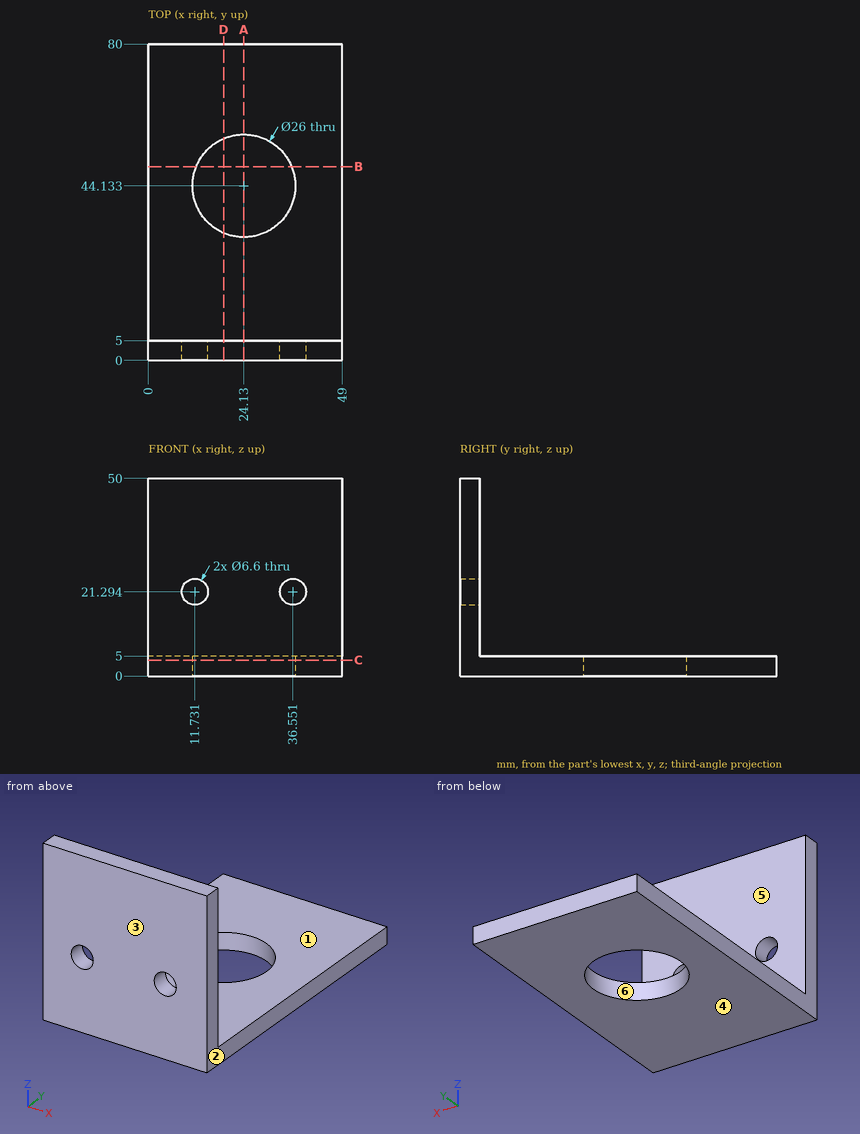
Part print with two shaded views. Sizes in mm from the minimum x, y, z corner. A direction names the side the tool comes from. Round coordinates to 2 decimals unless told otherwise and drop trailing zeros. Order: outer loops, then holes, each group sorted by start corner. A loop starts at its lowest first (then second) coordinate and runs counter-clockwise, first axis right, second up.
(1) Band-saw the part on D-D (x = 19). List the corners of the cut face in (y, z).
(2) Band-saw the part on B-B (y = 49). List the corners of the cut face in (x, z) (1 decimal).
(3) 3-axis set-ups, long thin cutter, end or side, ignore diameter. For the marked faces 1 and 2: which of +Z, -Z, +X, -X, +Y, -Y reach the whole face in a straight line?
(4) Pull direction Y, two halves, no side cores. Call the marked faces 3, 4, 5 and 6: released by +Y, released by -Y, zero draft, split by the parting line, or undercut.
(5) Pin check, flat tips, straight feed: pin 1 (14.5 mm diameter, centred on x = 17.5, y = 31, fed in from +Z); pin 2 (7.5 mm diameter, centred on x = 11.73, z = 21.29, fed in from +Y). Stop position of each tip, or through.
(6) Band-saw the part on C-C (z = 4). List the corners of the cut face in (x, y), then the cut area to 3 significant figures.
(7) Drill centre lines: line 1 (Y direction, x = 24, z = 3); line 2 (Z direction, x = 26, y = 14). Where is each one in solid material? Low to high.
(8) Band-saw the part on A-A (x = 24.13). List the corners of the cut face in (y, z), then the cut area to 3 significant figures.
Verdict:
1. outline: (0, 0) - (32.19, 0) - (32.19, 5) - (5, 5) - (5, 50) - (0, 50) - close; (56.08, 0) - (80, 0) - (80, 5) - (56.08, 5) - close
2. outline: (0, 0) - (12.1, 0) - (12.1, 5) - (0, 5) - close; (36.2, 0) - (49, 0) - (49, 5) - (36.2, 5) - close
3. face 1: +Z, +X, -X, +Y
3. face 2: +Z, -Z, +X, +Y, -Y
4. face 3: released by -Y
4. face 4: zero draft
4. face 5: released by +Y
4. face 6: undercut
5. pin 1: stops at z = 5
5. pin 2: stops at y = 5
6. outline: (0, 0) - (49, 0) - (49, 80) - (0, 80) - close; hole circle Ø26 at (24.13, 44.13)
6. area: 3,390 mm2
7. line 1: y = 0 to 31.13, 57.13 to 80
7. line 2: z = 0 to 5
8. outline: (0, 0) - (31.13, 0) - (31.13, 5) - (5, 5) - (5, 50) - (0, 50) - close; (57.13, 0) - (80, 0) - (80, 5) - (57.13, 5) - close
8. area: 495 mm2
